Check sheet for the drawn part. Datum: minimum x, y, z corner. Units: mm. Coordinates: 2 decimals unless noted, no trailing zeros. Write each loop counter-clockwise with the first axis right and the second up, starting at its lowest first coordinate (ties: lowest second). Pieces come first, ordered by that corner, then holes. Notation, with made-up numbers: (22, 34.5) -> (39, 34.5) arc R29 ccw to (39, 63.5) -> close; hole circle Ø9 at (-25, 72). An arc over 180 degrees is marked (long way). Answer in a Markdown table with one row per item. Add a question column.
1. Scan lines: L1, parallel to Z at x = 110, y = 4; L2, parallel to Z at x = 82, y = 1; L3, parallel to Z at x = 230, y = 1.75. Record each from-to range of solid material in increasing order. Write a range as from..to.
2. Cross-section at A-A on x = 239. Record the cut outline in (y, z).
3. Cross-section at B-B on z = 135. Record the cut outline in (x, y).
4. Cross-section at C-C on y = 1.5. Record the cut outline in (x, z).
5. Cross-section at D-D on x = 190. Record the cut outline in (y, z), and give its area (3 significant figures).
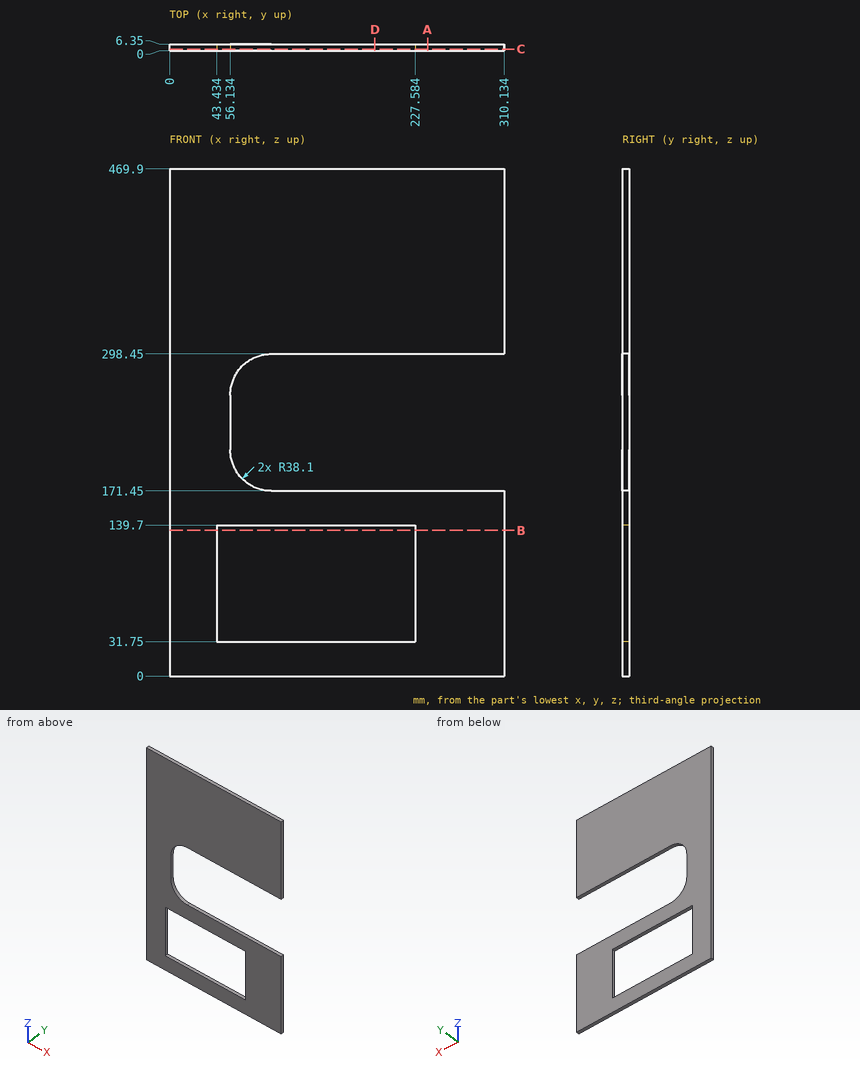
Results found:
| question | item | result |
|---|---|---|
| 1 | L1 | z = 0..31.75, 139.7..171.45, 298.45..469.9 |
| 1 | L2 | z = 0..31.75, 139.7..173.47, 296.43..469.9 |
| 1 | L3 | z = 0..171.45, 298.45..469.9 |
| 2 | outline | (0, 0) -> (6.35, 0) -> (6.35, 171.45) -> (0, 171.45) -> close; (0, 298.45) -> (6.35, 298.45) -> (6.35, 469.9) -> (0, 469.9) -> close |
| 3 | outline | (0, 0) -> (43.43, 0) -> (43.43, 6.35) -> (0, 6.35) -> close; (227.58, 0) -> (310.13, 0) -> (310.13, 6.35) -> (227.58, 6.35) -> close |
| 4 | outline | (0, 0) -> (310.13, 0) -> (310.13, 171.45) -> (94.23, 171.45) arc R38.1 cw to (56.13, 209.55) -> (56.13, 260.35) arc R38.1 cw to (94.23, 298.45) -> (310.13, 298.45) -> (310.13, 469.9) -> (0, 469.9) -> close; hole (43.43, 31.75) -> (227.58, 31.75) -> (227.58, 139.7) -> (43.43, 139.7) -> close |
| 5 | outline | (0, 0) -> (6.35, 0) -> (6.35, 31.75) -> (0, 31.75) -> close; (0, 139.7) -> (6.35, 139.7) -> (6.35, 171.45) -> (0, 171.45) -> close; (0, 298.45) -> (6.35, 298.45) -> (6.35, 469.9) -> (0, 469.9) -> close |
| 5 | area | 1,490 mm^2 |
